The figure shows three views and two pictorial views of one solid part (mm, origin at its lowest corner). Answer the questions. A direction names the side the tool comes from. Coordinates: 2 decimals unless noted, no trailing zeros. Order: outer loops, then holes, each group sorted by start corner. A loop starts at its lowest first (then second) coordinate and runs counter-clockwise, first axis right, second up.
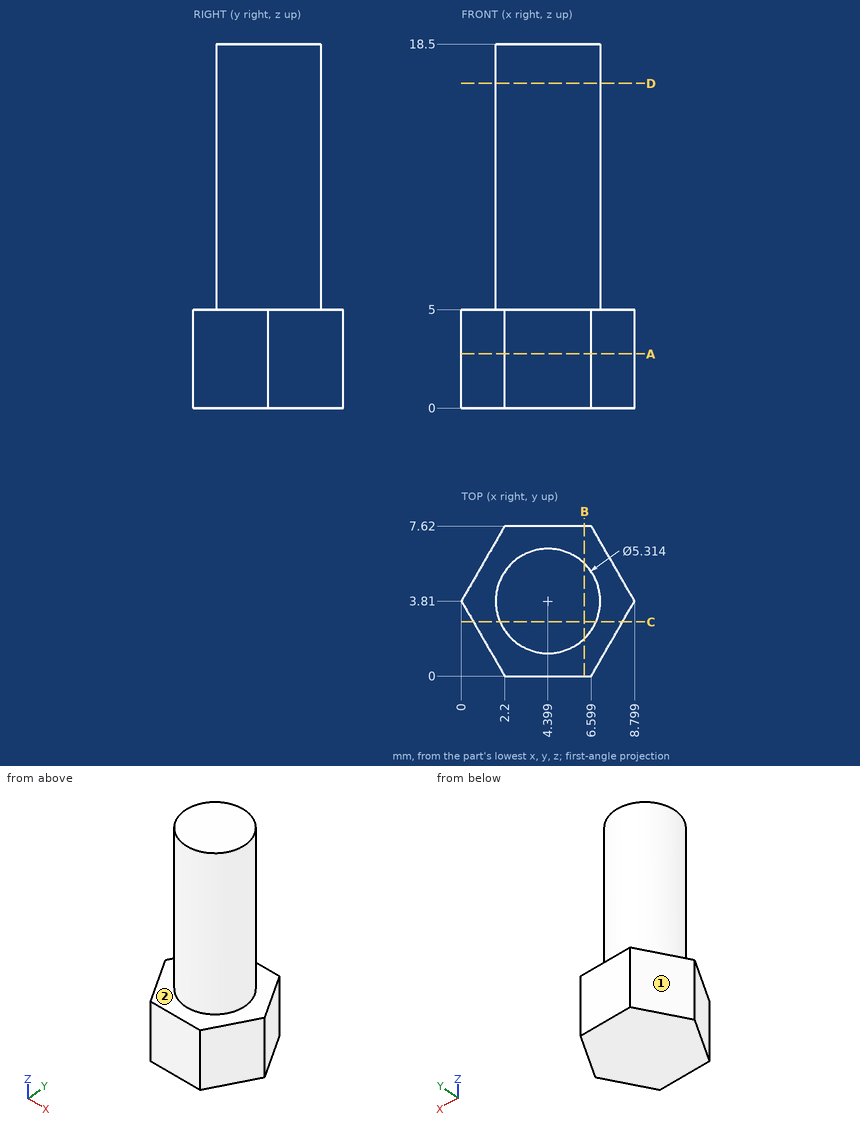
1) For the marked faces 1 and 2, determine the directions among +Z, -Z, +X, -X, +Y, -Y from which every point of the face is accessible in a straight line to the end or side of a thin tool.
2) A cutting plane is placed at D-D, the plane z = 16.5. Write down the section's boundary in (x, y).
3) A cutting plane is placed at B-B, the plane x = 6.25. Write down the section's boundary in (y, z).
4) A cutting plane is placed at A-A, the plane z = 2.75. Write down the section's boundary in (x, y).
5) Each of these flat-tipped pins is pushed along its axis until it touches: P1, Ø1, axis at y = 5, z = 6, coming from the -X side; P2, Ø2, axis at x = 4, z = 6.5, coming from the -Y side. Where does it stop, or does it pass through?
6) A cutting plane is placed at C-C, the plane y = 2.75. Write down the section's boundary in (x, z) (1 decimal).
7) Straight lines are drawn through the part: probe 1 along Z at (x, y) = (1.5, 4); probe 2 along X at (y, z) = (3.75, 16) (1 decimal); probe 3 along X at (y, z) = (5.5, 1.25) (1 decimal). For each, find the intervals that lie inside material, in ascending order.
Working result:
1. face 1: +Z, -Z, -X, +Y
1. face 2: +Z
2. outline: circle Ø5.31 at (4.4, 3.81)
3. outline: (0, 0) - (7.62, 0) - (7.62, 5) - (5.72, 5) - (5.72, 18.5) - (1.9, 18.5) - (1.9, 5) - (0, 5) - close
4. outline: (0, 3.81) - (2.2, 0) - (6.6, 0) - (8.8, 3.81) - (6.6, 7.62) - (2.2, 7.62) - close
5. P1: stops at x = 1.83
5. P2: stops at y = 1.15
6. outline: (0.6, 0) - (8.2, 0) - (8.2, 5) - (6.8, 5) - (6.8, 18.5) - (2, 18.5) - (2, 5) - (0.6, 5) - close
7. probe 1: z = 0 to 5
7. probe 2: x = 1.7 to 7.1
7. probe 3: x = 1 to 7.8
